Autodesk Inventor part; units mm, degrees
ref_plane "YZ Plane" through (0, 0, 0) normal (1, 0, 0) x (0, 1, 0)
ref_plane "XZ Plane" through (0, 0, 0) normal (0, 1, 0) x (-1, 0, 0)
ref_plane "XY Plane" through (0, 0, 0) normal (0, 0, 1) x (1, 0, 0)
sketch "Sketch9" plane through (0, 0, 0) normal (0, 0, 1) x (1, 0, 0)
  line L0 (0, 0) -> (0, 55) construction
  circle A0 centre (0, 55) radius 1.5
  circle A1 centre (0, 0) radius 1.5
  circle A2 centre (0, 27.5) radius 1.5
  line L1 (-10, 60) -> (10, 60)
  line L2 (10, 60) -> (10, -5)
  line L3 (10, -5) -> (-10, -5)
  line L4 (-10, -5) -> (-10, 60)
  point P0 (-10, 27.5)
  point P1 (0, 60)
  dimension "d35" = 55
  dimension "d36" = 3
  dimension "d37" = 3
  dimension "d38" = 3
  dimension "d39" = 5
  dimension "d40" = 10
extrude "Extrusion9" add sketch "Sketch9" along normal blind 10
sketch "Sketch11" plane through (10, -5, 0) normal (1, 0, 0) x (0, 0, -1)
  line L0 (0, 65) -> (-10, 65)
  line L1 (0, 65) -> (-75, 65)
  line L2 (-75, 65) -> (-75, 50)
  line L3 (-75, 50) -> (0, 50)
  line L4 (0, 50) -> (0, 65)
  point P0 (0, 5)
  dimension "d43" = 15
  dimension "d44" = 75
extrude "Extrusion10" add sketch "Sketch11" along normal blind 35
sketch "Sketch12" plane through (-10, 60, 10) normal (0, 1, 0) x (1, 0, 0)
  line L0 (20, -65) -> (20, 0)
  line L1 (20, -65) -> (34, -65)
  line L2 (34, -65) -> (34, 0)
  line L3 (34, 0) -> (20, 0)
  line L4 (20, 0) -> (20, -65)
  point P0 (10, 10)
  dimension "d47" = 14
extrude "Extrusion11" cut sketch "Sketch12" against normal through all
chamfer "Chamfer6" distance 14 angle 45 1 edges at (24, 52.5, 10)
sketch "Sketch14" plane through (10, 45, 0) normal (0, -1, 0) x (1, 0, 0)
  line L0 (0, 10) -> (14, 24)
  line L1 (15.4558, 0) -> (35, 19.5442)
  line L2 (35, 75) -> (35, 0)
  line L3 (0, 0) -> (35, 0)
  line L4 (15.4558, 0) -> (35, 0)
  line L5 (35, 19.5442) -> (35, 0)
  point P0 (-10, 0)
  dimension "d73" = 18
extrude "Extrusion13" cut sketch "Sketch14" against normal through all
sketch "Sketch15" plane through (0, 0, 0) normal (0, 0, -1) x (-1, 0, 0)
  line L0 (-25.4558, 60) -> (-25.4558, 45)
  line L1 (-10, 45) -> (-25.4558, 45)
  line L2 (-10, 45) -> (-10, -5)
  line L3 (-10, -5) -> (10, -5)
  line L4 (10, -5) -> (10, 60)
  line L5 (10, 60) -> (-25.4558, 60)
  circle A0 centre (0, 55) radius 1.5
  circle A1 centre (0, 0) radius 1.5
  circle A2 centre (0, 27.5) radius 1.5
  line L6 (-10, -5) -> (10, -5)
  line L7 (10, 60) -> (-10, 60)
  line L8 (-10, -5) -> (-10, 60)
  line L9 (-10, 60) -> (10, 60)
extrude "Extrusion14" add sketch "Sketch15" along normal blind 3 contours L5 L4 L3 L2 L8
chamfer "Chamfer8" distance 3 angle 45 1 edges at (-10, 27.5, 10)
equation "\"Module\" = 2"
equation "\"PressureAngle\" = 20deg"
equation "\"UnitProfileClearance\" = 0.25"
equation "\"UnitRoundRadius\" = 0.35"
equation "\"HeadDiameter\" = 42"
equation "\"RootDiameter\" = 33"
equation "\"BaseDiameter\" = 35.70832"
equation "\"PitchDiameter\" = 38"
equation "\"HelixAngle\" = 0"
equation "\"UnitCorrection\" = 0"
equation "\"UnitAddendumModification\" = 0"
equation "\"CircularPitch\" = 6.283185"
equation "\"UnitBacklashShift\" = 0"
equation "\"TotalToolShift\" = 0"
equation "\"IsInternal\" = 0"
properties part number "GA04" material "ABS Plastic"
Verification items for the finished model (mm, model axes). A direction names the side the tool comes from. Give positions to 0.01 mm unless a question says otherwise; leave off trailing zeros. Loops run counter-clockwise (first coordinate to the right, second up) from the corner with the lowest first, then second, coordinate; pieces in that order, holes last. Notation, with made-up numbers: (-8, -9) - (49, -9) arc R22 cw to (49, 16) - close; hole circle Ø6 at (83.25, -29.75). An arc over 180 degrees is marked (long way). Write item = value, one per line. Start each with the question number.
Q1. Cross-section at D-D, the plane y = 43.5. Enter the section's corners in (x, z).
Q2. Cross-section at B-B, the plane y = 0. Enter the section's corners in (x, z), and give its area (4 significant figures).
Q3. Tool access check on faces 1 (the face through (18, 53, 0)), 2 (the face through (24, 53, 50)), 3 (the face through (0, -5, 4)). Record the directions out of +Z, -Z, +X, -X, +Y, -Y that give a thin tool (end or side, any length) a straight path to the whole face; none if there is none.
Q4. Cross-section at C-C, the plane z = 4.5. Enter the section's corners in (x, y).
Q5. Cross-section at A-A, the plane x = 0. Enter the section's corners in (y, z).
Q6. Depth check by flat-ended pin: P1, Ø10.5, axis at y = 42, z = 4.5, coming from the +X side; P2, Ø4, axis at x = 0, y = 0, coming from the +Z side; P3, Ø1.8, axis at x = 0, y = 55, coming from the +Z side; P4, Ø12, axis at x = 37.5, z = 47.5, coming from the -Y side. Enter the tip coordinate at first touch or a pass-through.
Q7. Thickness scan on line 1 (Y direction, x = 0, z = -0.9); line 2 (X direction, y = 55, z = -0.7); line 3 (Z direction, x = 5, y = 26). Record the ranges inside material, lowest first.
Answer key:
q1.outline = (-10, -3) - (10, -3) - (10, 10) - (-7, 10) - (-10, 7) - close
q2.outline = (-10, -3) - (-1.5, -3) - (-1.5, 10) - (-7, 10) - (-10, 7) - close; (1.5, -3) - (10, -3) - (10, 10) - (1.5, 10) - close
q2.area = 216.5 mm^2
q3.face_1 = -Z, +X, +Y, -Y
q3.face_2 = +Z, -X, +Y, -Y
q3.face_3 = +Z, -Z, +X, -X, -Y
q4.outline = (-10, -5) - (10, -5) - (10, 45) - (29.96, 45) - (29.96, 60) - (-10, 60) - close; hole circle Ø3 at (0, 0); hole circle Ø3 at (0, 27.5); hole circle Ø3 at (0, 55)
q5.outline = (-5, -3) - (-1.5, -3) - (-1.5, 10) - (-5, 10) - close; (1.5, -3) - (26, -3) - (26, 10) - (1.5, 10) - close; (29, -3) - (53.5, -3) - (53.5, 10) - (29, 10) - close; (56.5, -3) - (60, -3) - (60, 10) - (56.5, 10) - close
q6.P1 = 34.26
q6.P2 = 10
q6.P3 = through
q6.P4 = 45
q7.line_1 = -5 to -1.5, 1.5 to 26, 29 to 53.5, 56.5 to 60
q7.line_2 = -10 to -1.5, 1.5 to 10
q7.line_3 = -3 to 10
